Check sheet for the modelled part. Datum: model origin and axes. Units: mm. Face numbers are marked on the shaded views. A direction names the side the tool comes from. Give positions to 0.01 mm unless a question says otherwise; leave off trailing zeros. Loops run counter-clockwise (first coordinate to the right, second up) from the corner with the lowest first, then second, coordinate; pieces in that order, holes last. Notation, with made-up numbers: (11, 7.25) -> (64, 7.25) arc R30 ccw to (64, 31.25) -> close; hole circle Ø4 at (82.5, 84.5). An arc over 180 degrees is marked (long way). Answer as CSV lines item,"result". Start each with the question number.
(1) Section check C-C on z = 5.5. Enter the section's corners in (x, y).
(2) Release check for a two-part mould opening along Z. For the marked faces 1, 2 and 3 record: pulls with the +Z half, pulls with the -Z half, needs draft (parallel to the pull), parting line crosses it, or undercut.
(3) Section check A-A on y = 15.5. Enter the section's corners in (x, z) (3 decimals), plus the area to 3 significant figures.
(4) Gauge pin test, flat ends, axial feed: pin 1 Ø8 at (x, y) = (-11, 12.5) entering from -Z; pin 2 Ø3 at (y, z) = (11, -30.5) entering from +X; pin 3 Ø12 at (y, z) = (2.5, 13) entering from +X. Record the tip position at first contact, or that the pin passes through.
(5) Section check B-B on x = 0. State how many separate pieces and enclosed holes the cut face has, plus the area to 3 significant figures.
(6) Access from +Z, -Z, +X, -X, +Y, -Y to the whole of each face (thin tool, end or side, straight path). Record for the marked faces 4, 5, 6, 7 and 8.
(7) Section check D-D on y = 11.5. Enter the section's corners in (x, z) (3 decimals), plus the area to 3 significant figures.
(8) Material ranges on line 1 (Z direction, x = 0, y = 13); line 2 (Z direction, x = 0, y = 3.45); line 3 (X direction, y = 6, z = 38.5), recorded low to high. Write a range as from..to.
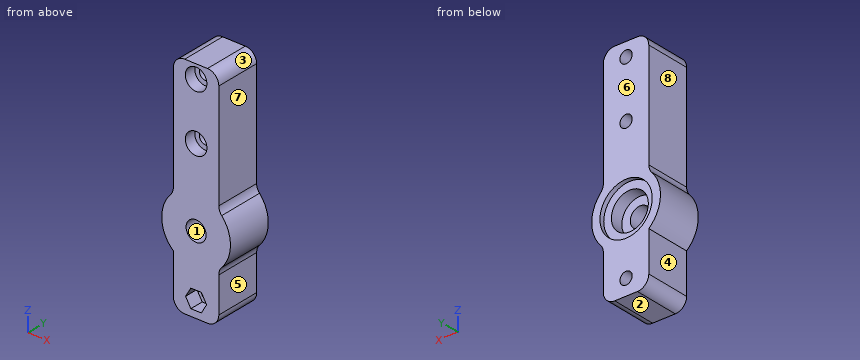
Autodesk Inventor part; units mm, degrees
ref_plane "YZ Plane" through (0, 0, 0) normal (1, 0, 0) x (0, 1, 0)
ref_plane "XZ Plane" through (0, 0, 0) normal (0, 1, 0) x (-1, 0, 0)
ref_plane "XY Plane" through (0, 0, 0) normal (0, 0, 1) x (1, 0, 0)
sketch "Boceto1" plane through (0, 0, 0) normal (0, 1, 0) x (-1, 0, 0)
  line L0 (-10, 44.5408) -> (10, 44.5408)
  line L1 (10, 44.5408) -> (10, -27.9592)
  line L2 (10, -27.9592) -> (-10, -27.9592)
  line L3 (-10, -27.9592) -> (-10, 44.5408)
  line L4 (-10, 44.5408) -> (10, -27.9592) construction
  line L5 (10, 44.5408) -> (-10, -27.9592) construction
  circle A0 centre (0, -20.4592) radius 4.4
  point P0 (0, 8.2908)
  dimension "d1" = 20
  dimension "d2" = 8.8
  dimension "d3" = 7.5
  dimension "d26" = 65
extrude "Extrusión1" add sketch "Boceto1" along normal blind 20
sketch "Boceto2" plane through (0, 20, 0) normal (0, 1, 0) x (1, 0, 0)
  circle A0 centre (0, 20.4592) radius 4.4
  circle A1 centre (0, 20.4592) radius 12.125
  point P0 (0, 0)
  dimension "d6" = 24.25
extrude "Extrusión2" cut sketch "Boceto2" against normal blind 2.5
sketch "Boceto3" plane through (0, 20, 0) normal (0, 1, 0) x (1, 0, 0)
  circle A0 centre (0, 20.4592) radius 4.4
  circle A1 centre (0, 20.4592) radius 12.125
  circle A2 centre (0, 20.4592) radius 15.125
  line L0 (10, 27.316) -> (10, 13.6024)
  arc A3 (10, 27.316) -> (9.5271, 27.9592) centre (0, 20.4592) ccw
  line L1 (-9.5271, 27.9592) -> (9.5271, 27.9592)
  arc A4 (-9.5271, 27.9592) -> (-10, 27.316) centre (0, 20.4592) ccw
  line L2 (-10, 13.6024) -> (-10, 27.316)
  arc A5 (-10, 13.6024) -> (10, 13.6024) centre (0, 20.4592) ccw
  circle A6 centre (0, 20.4592) radius 4.4
  point P0 (0, 0)
  point P1 (-10, 27.316)
  point P2 (10, 27.316)
  point P3 (9.5271, 27.9592)
  dimension "d9" = 3
extrude "Extrusión3" add sketch "Boceto3" against normal up to surface (20 mm away) contours A1 L0 | L1 A1 | A1 L2 | A2
sketch "Boceto4" plane through (0, 20, 0) normal (0, 1, 0) x (1, 0, 0)
  circle A0 centre (0, 20.4592) radius 4.4
  circle A1 centre (0, 20.4592) radius 12.15
  point P0 (0, 0)
  dimension "d14" = 24.3
extrude "Extrusión4" cut sketch "Boceto4" against normal blind 2 contours A0 | A1
sketch "Boceto5" plane through (0, 17.5, 0) normal (0, 1, 0) x (1, 0, 0)
  line L0 (10, 27.316) -> (10, 13.6024)
  arc A0 (10, 27.316) -> (9.5271, 27.9592) centre (0, 20.4592) ccw
  line L1 (-9.5271, 27.9592) -> (9.5271, 27.9592)
  arc A1 (-9.5271, 27.9592) -> (-10, 27.316) centre (0, 20.4592) ccw
  line L2 (-10, 13.6024) -> (-10, 27.316)
  arc A2 (-10, 13.6024) -> (10, 13.6024) centre (0, 20.4592) ccw
  circle A3 centre (0, 20.4592) radius 4.4
  point P0 (0, 0)
extrude "Extrusión5" add sketch "Boceto5" along normal up to surface (0.5 mm away)
sketch "Boceto6" plane through (0, 0, 0) normal (0, -1, 0) x (1, 0, 0)
  circle A0 centre (0, 38.5408) radius 2.7
  circle A1 centre (0, 13.5408) radius 2.7
  line L0 (-10, 44.5408) -> (10, 44.5408)
  point P0 (0, 0)
  dimension "d20" = 25
  dimension "d21" = 5.4
  dimension "d30" = 6
extrude "Extrusión6" cut sketch "Boceto6" against normal through all
sketch "Boceto8" plane through (0, 18, -20.4592) normal (0, 1, 0) x (1, 0, 0)
  circle A0 centre (0, 0) radius 4.4
  circle A1 centre (0, 0) radius 8.125
  point P0 (0, -20.4592)
  dimension "d31" = 16.25
extrude "Extrusión8" cut sketch "Boceto8" against normal blind 5.5 contours A0 | A1
fillet "Empalme4" radius 5 4 edges at (10, 10, 44.5408) (-10, 10, 44.5408) (10, 10, -9.1117) (-10, 10, -9.1117)
sketch "Boceto9" plane through (0, 20, 0) normal (0, 1, 0) x (1, 0, 0)
  arc A0 (11.2733, 10.3756) -> (-11.2733, 10.3756) centre (0, 20.4592) ccw
  line L0 (-10, 31.8067) -> (10, 31.8067)
  line L1 (10, 31.8067) -> (10, 54.4592)
  line L2 (10, 54.4592) -> (-10, 54.4592)
  line L3 (-10, 54.4592) -> (-10, 31.8067)
  line L4 (-10, 7.0422) -> (-10, -39.5408)
  line L5 (10, -39.5408) -> (10, 7.0422)
  circle A1 centre (0, 20.4592) radius 21
  circle A2 centre (0, 47.4592) radius 2.7
  point P0 (0, 0)
  dimension "d36" = 42
  dimension "d37" = 34
  dimension "d38" = 5.4
  dimension "d39" = 7
extrude "Extrusión9" add sketch "Boceto9" against normal up to surface (20 mm away) contours A0 L3 A1 L1 | A1 L3 L2 L1
fillet "Empalme5" radius 5 3 edges at (10, 10, -31.8067) (10, 10, -54.4592) (-10, 10, -54.4592)
sketch "Boceto10" plane through (0, 0, 0) normal (0, -1, 0) x (1, 0, 0)
  circle A0 centre (0, -47.4592) radius 2.7
  circle A1 centre (0, -47.4592) radius 4
  line L0 (-4.6188, -47.4592) -> (-2.3094, -43.4592)
  line L1 (-2.3094, -43.4592) -> (2.3094, -43.4592)
  line L2 (2.3094, -43.4592) -> (4.6188, -47.4592)
  line L3 (4.6188, -47.4592) -> (2.3094, -51.4592)
  line L4 (2.3094, -51.4592) -> (-2.3094, -51.4592)
  line L5 (-2.3094, -51.4592) -> (-4.6188, -47.4592)
  point P0 (0, 6.5408)
  dimension "d43" = 8
extrude "Extrusión10" cut sketch "Boceto10" against normal blind 6 contours A0 | A1 | A1 L2 L3 | A1 L1 L2 | L3 L4 A1 | A1 L0 L1 | L4 L5 A1 | A1 L5 L0
sketch "Boceto11" plane through (0, 0, 0) normal (0, -1, 0) x (1, 0, 0)
  circle A0 centre (0, 38.5408) radius 2.7
  circle A1 centre (0, 38.5408) radius 4.75
  circle A2 centre (0, 13.5408) radius 2.7
  circle A3 centre (0, 13.5408) radius 4.75
  point P0 (0, 0)
  dimension "d46" = 9.5
  dimension "d47" = 9.5
extrude "Extrusión11" cut sketch "Boceto11" against normal blind 5
sketch "Boceto12" plane through (0, 20, 0) normal (0, 1, 0) x (1, 0, 0)
  circle A0 centre (0, 20.4592) radius 8.125
  circle A1 centre (0, 20.4592) radius 8.125
  circle A2 centre (0, 20.4592) radius 12.15
  point P0 (0, 0)
extrude "Extrusión12" add sketch "Boceto12" against normal up to surface (2 mm away)
sketch "Boceto14" plane through (0, 20, 0) normal (0, 1, 0) x (1, 0, 0)
  circle A0 centre (0, 20.4592) radius 8.125
  circle A1 centre (0, 20.4592) radius 11.5
  point P0 (0, 0)
  dimension "d55" = 23
extrude "Extrusión14" cut sketch "Boceto14" against normal blind 2
sketch "Boceto13" plane through (0, 12.5, -20.4592) normal (0, 1, 0) x (1, 0, 0)
  circle A0 centre (0, 0) radius 4.4
  circle A1 centre (0, 0) radius 8.125
  point P0 (0, -20.4592)
properties part number "bottomsupport"
Working result:
1,outline,"(-10, 0) -> (10, 0) -> (10, 20) -> (-10, 20) -> close"
2,face 1,"undercut"
2,face 2,"pulls with the -Z half"
2,face 3,"pulls with the +Z half"
3,outline,"(-11.273, -10.376) arc R15.125 ccw to (-10, -31.807) -> (-10, -49.459) arc R5 ccw to (-5, -54.459) -> (5, -54.459) arc R5 ccw to (10, -49.459) -> (10, -33.876) arc R5 cw to (11.273, -30.543) arc R15.125 ccw to (11.273, -10.376) arc R5 cw to (10, -7.042) -> (10, 39.541) arc R5 ccw to (5, 44.541) -> (-5, 44.541) arc R5 ccw to (-10, 39.541) -> (-10, -7.042) arc R5 cw to start; hole circle Ø16.25 at (0, -20.459); hole circle Ø5.4 at (0, -47.459); hole circle Ø5.4 at (0, 13.541); hole circle Ø5.4 at (0, 38.541)"
3,area,"1,850 mm^2"
4,pin 1,"stops at z = -54.04"
4,pin 2,"stops at x = 12.48"
4,pin 3,"stops at x = 10"
5,separate pieces,"5"
5,enclosed holes,"0"
5,area,"1,350 mm^2"
6,face 4,"-Z, -X, +Y, -Y"
6,face 5,"-Z, +X, +Y, -Y"
6,face 6,"+Z, -Z, +X, -X, +Y"
6,face 7,"+Z, +X, +Y, -Y"
6,face 8,"+Z, -X, +Y, -Y"
7,outline,"(-11.273, -10.376) arc R15.125 ccw to (-10, -31.807) -> (-10, -49.459) arc R5 ccw to (-5, -54.459) -> (5, -54.459) arc R5 ccw to (10, -49.459) -> (10, -33.876) arc R5 cw to (11.273, -30.543) arc R15.125 ccw to (11.273, -10.376) arc R5 cw to (10, -7.042) -> (10, 39.541) arc R5 ccw to (5, 44.541) -> (-5, 44.541) arc R5 ccw to (-10, 39.541) -> (-10, -7.042) arc R5 cw to start; hole circle Ø8.8 at (0, -20.459); hole circle Ø5.4 at (0, -47.459); hole circle Ø5.4 at (0, 13.541); hole circle Ø5.4 at (0, 38.541)"
7,area,"1,990 mm^2"
8,line 1,"z = -54.46..-50.16, -44.76..-28.58, -12.33..10.84, 16.24..35.84, 41.24..44.54"
8,line 2,"z = -54.46..-51.46, -43.46..-24.86, -16.06..8.79, 18.29..33.79, 43.29..44.54"
8,line 3,"x = -10..-2.7, 2.7..10"
